Autodesk Inventor part; units mm, degrees
ref_plane "YZ Plane" through (0, 0, 0) normal (1, 0, 0) x (0, 1, 0)
ref_plane "XZ Plane" through (0, 0, 0) normal (0, 1, 0) x (-1, 0, 0)
ref_plane "XY Plane" through (0, 0, 0) normal (0, 0, 1) x (1, 0, 0)
sketch "Sketch1" plane through (0, 0, 0) normal (0, 1, 0) x (-1, 0, 0)
  line L0 (50.8, 38.1) -> (-50.8, 38.1)
  line L1 (-50.8, 38.1) -> (-50.8, -38.1)
  line L2 (-50.8, -38.1) -> (50.8, -38.1)
  line L3 (50.8, -38.1) -> (50.8, 38.1)
  line L4 (50.8, 38.1) -> (-50.8, -38.1) construction
  line L5 (-50.8, 38.1) -> (50.8, -38.1) construction
  point P0 (0, 0)
  dimension "d0" = 76.2
  dimension "d1" = 101.6
extrude "Extrusion1" add sketch "Sketch1" along normal blind 6.35
sketch "Sketch2" plane through (0, 6.35, 0) normal (0, 1, 0) x (1, 0, 0)
  line L0 (25.4, -12.7) -> (25.4, 12.7)
  line L1 (25.4, 12.7) -> (-25.4, 12.7)
  line L2 (-25.4, 12.7) -> (-25.4, -12.7)
  line L3 (-25.4, -12.7) -> (25.4, -12.7)
  line L4 (25.4, -12.7) -> (-25.4, 12.7) construction
  line L5 (25.4, 12.7) -> (-25.4, -12.7) construction
  line L6 (22.225, -9.525) -> (22.225, 9.525)
  line L7 (22.225, 9.525) -> (-22.225, 9.525)
  line L8 (-22.225, 9.525) -> (-22.225, -9.525)
  line L9 (-22.225, -9.525) -> (22.225, -9.525)
  line L10 (22.225, -9.525) -> (-22.225, 9.525) construction
  line L11 (22.225, 9.525) -> (-22.225, -9.525) construction
  point P0 (0, 0)
  dimension "d4" = 50.8
  dimension "d5" = 25.4
  dimension "d6" = 3.175
  dimension "d7" = 3.175
extrude "Extrusion2" add sketch "Sketch2" along normal blind 152.4
sketch "Sketch5" plane through (0, 6.35, 0) normal (0, 1, 0) x (1, 0, 0)
  line L0 (-51.0645, -25.4) -> (50.8, -25.4) construction
  line L1 (50.8, -38.1) -> (50.8, 38.1) construction
  line L2 (-38.1, -38.1) -> (-38.1, 38.1) construction
  line L3 (50.8, 38.1) -> (-50.8, 38.1) construction
  line L4 (-50.8, -38.1) -> (50.8, -38.1) construction
  line L5 (-50.8, 38.1) -> (-50.8, -38.1) construction
  point P0 (0, 0)
  point P1 (-38.1, -25.4)
  point P2 (-12.7, -25.4)
  point P3 (12.7, -25.4)
  point P4 (38.1, -25.4)
  point P5 (-38.1, 0)
  point P6 (-12.7, 0)
  point P7 (12.7, 0)
  point P8 (38.1, 0)
  point P9 (-38.1, 25.4)
  point P10 (-12.7, 25.4)
  point P11 (12.7, 25.4)
  point P12 (38.1, 25.4)
  dimension "d19" = 12.7
  dimension "d20" = 12.7
  dimension "d23" = 25.4
  dimension "d26" = 25.4
hole "Hole2" at (-38.1, 6.35, 25.4) at (-12.7, 6.35, 25.4) at (12.7, 6.35, 25.4) at (38.1, 6.35, 25.4) at (-38.1, 6.35, 0) at (-12.7, 6.35, 0) at (12.7, 6.35, 0) at (38.1, 6.35, 0) at (-38.1, 6.35, -25.4) at (-12.7, 6.35, -25.4) at (12.7, 6.35, -25.4) at (38.1, 6.35, -25.4) direction (0, -1, 0) diameter 6.7564 end through all
sketch "Sketch6" plane through (-25.4, 6.35, 12.7) normal (0, 0, 1) x (1, 0, 0)
  line L0 (3.175, 0) -> (47.625, 0) construction
  line L1 (25.4, 0) -> (25.4, 152.4) construction
  line L2 (50.8, 152.4) -> (0, 152.4) construction
  line L3 (-1.017, 120.65) -> (50.8, 120.65) construction
  line L4 (50.8, 0) -> (50.8, 152.4) construction
  line L5 (-25.4, -6.35) -> (76.2, -6.35)
  point P0 (25.4, -6.35)
  point P1 (25.4, 120.65)
  dimension "d36" = 127
hole "Hole3" at (0, 127, 12.7) direction (0, 0, -1) diameter 28.575 end through all
properties part number "PostForHexAxel"
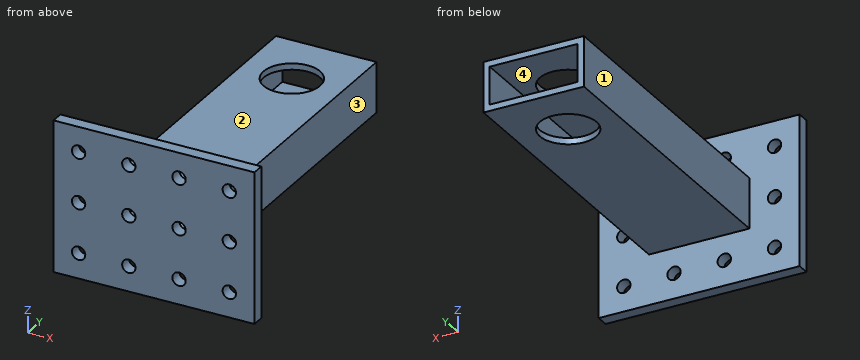
Here's how the part is built. I have some questions about the finished solid (model axes, mm). Face numbers are marked on the shaded views. A direction names the side the tool comes from. Round coordinates to 2 decimals unless told otherwise and drop trailing zeros. Write each loop counter-clockwise with the first axis right and the second up, starting at its lowest first coordinate (ties: lowest second). Pieces come first, ordered by that corner, then holes.
Q1. If we section it at A-A on z = -25.4: Write out the boundary of the cut face in (x, y), plus the area to 3 significant figures.
Q2. If we section it at B-B on x = 38.1: Write out the boundary of the cut face in (y, z), plus the area to 3 significant figures.
Q3. Please list where these lines run through material, in increasing order: probe 1 along X at (y, z) = (4, 25); probe 2 along Z at (x, y) = (38.1, 5.25); probe 3 along X at (y, z) = (77, -6.5) (3 decimals).
Q4. Which directions (+Z, -Z, +X, -X, +Y, -Y) give clear straight access to the entire face, cutting with the end or side of a thin tool? Please do the marked faces 1, 2, 3 and 4.
Q5. If we section it at D-D on x = 0: Give the number of separate pieces and of enclosed holes in the cut face, plus the area to 3 significant figures.
Q6. Will these pins go through, and if not, where does the flat tip stop? P1, Ø4, axis at x = -38.1, z = 25.4, coming from the +Y side; P2, Ø4, axis at y = 38, z = 7, coming from the -X side; P3, Ø10, axis at x = 5.5, z = -8, coming from the -Y side; P4, Ø11, axis at x = 38.1, z = 25.4, coming from the +Y side.
Q7. If we section it at C-C on y = 49.5: Write out the boundary of the cut face in (x, z) (3 decimals).
Answer below:
1. outline: (-50.8, 0) - (-41.48, 0) - (-41.48, 6.35) - (-50.8, 6.35) - close; (-34.72, 0) - (-16.08, 0) - (-16.08, 6.35) - (-34.72, 6.35) - close; (-9.32, 0) - (9.32, 0) - (9.32, 6.35) - (-9.32, 6.35) - close; (16.08, 0) - (34.72, 0) - (34.72, 6.35) - (16.08, 6.35) - close; (41.48, 0) - (50.8, 0) - (50.8, 6.35) - (41.48, 6.35) - close
1. area: 474 mm2
2. outline: (0, -38.1) - (6.35, -38.1) - (6.35, -28.78) - (0, -28.78) - close; (0, -22.02) - (6.35, -22.02) - (6.35, -3.38) - (0, -3.38) - close; (0, 3.38) - (6.35, 3.38) - (6.35, 22.02) - (0, 22.02) - close; (0, 28.78) - (6.35, 28.78) - (6.35, 38.1) - (0, 38.1) - close
2. area: 355 mm2
3. probe 1: x = -50.8 to -41.45, -34.75 to -16.05, -9.35 to 9.35, 16.05 to 34.75, 41.45 to 50.8
3. probe 2: z = -38.1 to -28.78, -22.02 to -3.38, 3.38 to 22.02, 28.78 to 38.1
3. probe 3: x = -25.4 to -22.225, 22.225 to 25.4
4. face 1: +Z, -Z, -X, +Y
4. face 2: +Z, +X, -X, +Y
4. face 3: +Z, -Z, +X, +Y
4. face 4: +Y
5. separate pieces: 3
5. enclosed holes: 0
5. area: 1,270 mm2
6. P1: passes through
6. P2: stops at x = -25.4
6. P3: stops at y = 0
6. P4: stops at y = 6.35
7. outline: (-25.4, -12.7) - (25.4, -12.7) - (25.4, 12.7) - (-25.4, 12.7) - close; hole (-22.225, -9.525) - (22.225, -9.525) - (22.225, 9.525) - (-22.225, 9.525) - close
